Geometry: final body of the model. Coordinates: model frame, mm. A direction names the side the tool comes from. Round coordinates to 2 decimals unless told otherwise and drop trailing zeros. Loops run counter-clockwise (first coordinate to the right, second up) from the corner with the lowest first, then second, coordinate; pieces in that order, holes last. Notation, with made-up numbers: (23.5, 56) -> (34.5, 56) arc R26 cw to (34.5, 90) -> close; hole circle Ø2 at (-12.75, 70). An arc over 180 degrees is marked (long way). Answer in a Markdown table with one row per item.
```python
from build123d import *

# Parameters (mm, degrees)
SKETCH1_R           = 17.145
SKETCH1_R_2         = 13.335
BOSS_EXTRUDE1_DEPTH = 84.328
SKETCH2_R           = 17.145
SKETCH2_R_2         = 13.335
BOSS_EXTRUDE2_DEPTH = 35.56
SKETCH3_R           = 13.335
CUT_EXTRUDE1_DEPTH  = 94.111096186
CUT_EXTRUDE2_START  = -35.56
SKETCH4_R           = 13.335
CUT_EXTRUDE2_DEPTH  = 35.56


with BuildPart() as part:
    # Sketch1 → Boss-Extrude1 (new body)
    with BuildSketch(Plane(origin=(0, 0, 0), x_dir=(1, 0, 0), z_dir=(0, 1, 0))):
        with Locations(Location((0, 0, 0), (0, 0, 270))):
            Circle(SKETCH1_R)
        with Locations(Location((0, 0, 0), (0, 0, 270))):
            Circle(SKETCH1_R_2, mode=Mode.SUBTRACT)
    extrude(amount=BOSS_EXTRUDE1_DEPTH)

    # Sketch2 → Boss-Extrude2 (add)
    with BuildSketch(Plane.XY):
        with Locations((0, 42.164)):
            Circle(SKETCH2_R)
        with Locations((0, 42.164)):
            Circle(SKETCH2_R_2, mode=Mode.SUBTRACT)
    extrude(amount=-BOSS_EXTRUDE2_DEPTH)

    # Sketch3 → Cut-Extrude1 (cut, through all)
    with BuildSketch(Plane(origin=(0, 84.328, 0), x_dir=(1, 0, 0), z_dir=(0, 1, 0))):
        with Locations(Location((0, 0, 0), (0, 0, 270))):
            Circle(SKETCH3_R)
    extrude(amount=-CUT_EXTRUDE1_DEPTH, mode=Mode.SUBTRACT)

    # Sketch4 → Cut-Extrude2 (cut)
    with BuildSketch(Plane(origin=(0, 0, -35.56), x_dir=(-1, 0, 0), z_dir=(0, 0, -1)).offset(CUT_EXTRUDE2_START)):
        with Locations(Location((0, 42.164, 0), (0, 0, 180))):
            Circle(SKETCH4_R)
    extrude(amount=CUT_EXTRUDE2_DEPTH, mode=Mode.SUBTRACT)


solid = part.part
```
Item 1: Line query: probe 1 along X at (y, z) = (32.5, 0) (3 decimals); probe 2 along Z at (x, y) = (0, 28) (3 decimals); probe 3 along Y at (x, z) = (0, -23). Output: solid intervals per line, ascending. Write a range as [from, to].
Answer:
| item | result |
|---|---|
| probe 1 | x = [-17.145, -13.335], [13.335, 17.145] |
| probe 2 | z = [-35.56, -13.335], [13.335, 17.145] |
| probe 3 | y = [25.02, 28.83], [55.5, 59.31] |
Item 2: Cut plane C-C (y = 39). Output: boundary loops of the cut face in (x, z) (3 decimals), then the cut area to 3 significant figures.
Answer:
| item | result |
|---|---|
| outline | (-16.851, -35.56) -> (-12.954, -35.56) -> (-12.954, -3.164) arc R13.335 cw (long way) to (12.954, -3.164) -> (12.954, -35.56) -> (16.851, -35.56) -> (16.851, -3.164) arc R17.145 ccw (long way) to (-16.851, -3.164) -> close |
| area | 459 mm² |
Item 3: Cut plane A-A (x = 0). Output: boundary loops of the cut face in (y, z) (3 decimals), then the cut area to 3 significant figures.
Answer:
| item | result |
|---|---|
| outline | (0, -17.145) -> (25.019, -17.145) -> (25.019, -35.56) -> (28.829, -35.56) -> (28.829, -13.335) -> (0, -13.335) -> close; (0, 13.335) -> (84.328, 13.335) -> (84.328, 17.145) -> (0, 17.145) -> close; (55.499, -35.56) -> (59.309, -35.56) -> (59.309, -17.145) -> (84.328, -17.145) -> (84.328, -13.335) -> (55.499, -13.335) -> close |
| area | 681 mm² |
Item 4: Pin query (flat end, axial travel): pin 1 Ø4 at (x, y) = (-2.5, 53) entering from -Z; pin 2 Ø5 at (x, y) = (-10, 53) entering from +Z; pin 3 Ø12 at (x, y) = (13, 16) entering from -Z. Return the tip coordinate at first contact, or that it passes through.
Answer:
| item | result |
|---|---|
| pin 1 | stops at z = 12.55 |
| pin 2 | stops at z = 15.42 |
| pin 3 | stops at z = -15.65 |
Item 5: Draft query along X for faces 3 (the face through (4.005, 41.574, 12.719)), 4 (the face through (-8.81, 0, -10.24)), 5 (the face through (5.15, 41.574, 16.353)). Return one class per face: pulls with the +X half, pulls with the -X half, needs draft (parallel to the pull), parting line crosses it, or undercut.
Answer:
| item | result |
|---|---|
| face 3 | undercut |
| face 4 | needs draft |
| face 5 | parting line crosses it |
Item 6: Cut plane B-B (z = -9.5). Output: boundary loops of the cut face in (x, y) (3 decimals), then the cut area to 3 significant figures.
Answer:
| item | result |
|---|---|
| outline | (-14.272, 0) -> (-9.358, 0) -> (-9.358, 32.664) arc R13.335 cw to (-9.358, 51.664) -> (-9.358, 84.328) -> (-14.272, 84.328) -> (-14.272, 51.664) arc R17.145 ccw to (-14.272, 32.664) -> close; (9.358, 0) -> (14.272, 0) -> (14.272, 32.664) arc R17.145 ccw to (14.272, 51.664) -> (14.272, 84.328) -> (9.358, 84.328) -> (9.358, 51.664) arc R13.335 cw to (9.358, 32.664) -> close |
| area | 799 mm² |
Item 7: Cut plane D-D (y = 21). Output: boundary loops of the cut face in (x, z) (3 decimals).
Answer:
| item | result |
|---|---|
| outline | circle Ø34.29 at (0, 0); hole circle Ø26.67 at (0, 0) |
Item 8: Reachability of faces 1 (the face through (-12.64, 53.75, -21.48)), 2 (the face through (-8.81, 84.328, -10.24)) from +Z, -Z, +X, -X, +Y, -Y: full face, straight path, thin tool, end or side. Return the list, or none.
Answer:
| item | result |
|---|---|
| face 1 | -Z |
| face 2 | +Z, -Z, +X, -X, +Y |
